from build123d import *

# Parameters (mm, degrees)
F0_W     = 30.4900507075
F0_H     = 16.8403594638
F0_R     = 3.175
F1_DEPTH = 25.4
F2_R     = 3.175
F3_DEPTH = 25.4
F4_DEPTH = 25.4


# Not quite as in the source:
# - a feature names something its author has since deleted; it is built from what else it names


with BuildPart() as f1:
    # F0 (on Front) → F1 (new body)
    with BuildSketch(Plane.XZ):
        Rectangle(F0_W, F0_H)
        with Locations((-7.6225126769, 0)):
            Circle(F0_R, mode=Mode.SUBTRACT)
        with Locations((7.6225126769, 0)):
            Circle(F0_R, mode=Mode.SUBTRACT)
        with Locations((-7.6225126769, 0)):
            Circle(F0_R)
        with Locations((7.6225126769, 0)):
            Circle(F0_R)
    extrude(amount=F1_DEPTH)

    # F2 (on face) → F3 (join)
    with BuildSketch(Plane(origin=(0, 0, 0), x_dir=(-1, 0, 0), z_dir=(0, 1, 0))):
        with Locations((10.1633502358, 0)):
            Circle(F2_R)
        with Locations((-10.1633502358, 0)):
            Circle(F2_R)
    extrude(amount=F3_DEPTH)

    # F4 (add): a face of the model
    f4_faces = [f1.faces().sort_by_distance(p)[0] for p in [
        (15.2450253537, -12.7, 0),
    ]]
    extrude(f4_faces, amount=F4_DEPTH)


solid = f1.part
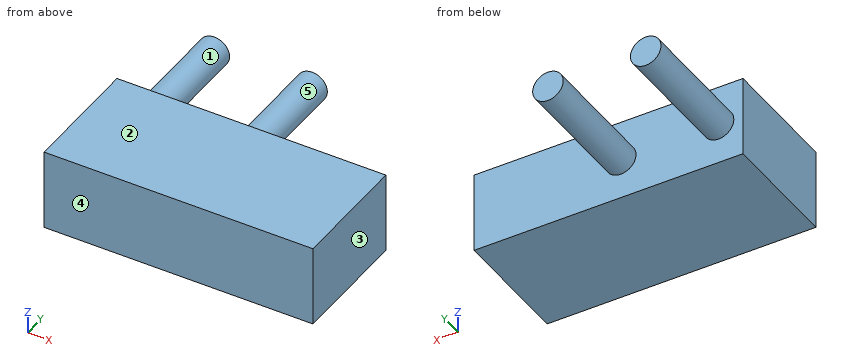
Check sheet for the modelled part. Datum: model origin and axes. Units: mm. Face numbers are marked on the shaded views. A direction names the side the tool comes from. Round coordinates to 2 decimals unless told otherwise and drop trailing zeros. Order: outer loops, then holes, each group sorted by start corner. A loop starts at its lowest first (then second) coordinate and runs counter-clockwise, first axis right, second up. Notation, with made-up numbers: M -7.75,-36.5 L 11.25,-36.5 A36 cw 11.25,1.5 Z; hole C 37,76 d8. An arc over 180 degrees is marked long. One line per item, written item: value. Start each with the question number.
1. Gauge pin test, flat ends, axial feed: P1, Ø12, axis at x = 15, y = 19.5, coming from the +Z side (3 decimals); P2, Ø3, axis at y = 19, z = 5.5, coming from the -X side; P3, Ø1, axis at y = 9.5, z = 3, coming from the -X side. Record the tip position at first contact, or that the pin passes through.
2. Scan lines: line 1 along Y through (x, z) = (-8, 5.25); line 2 along X through (y, z) = (2, -2.5); line 3 along X through (y, z) = (9, -0.5). Record each from-to range of solid material in increasing order.
3. Access from +Z, -Z, +X, -X, +Y, -Y to the whole of each face (thin tool, end or side, straight path). Record for the marked faces 1 and 2.
4. Section check A-A on z = 0. Enter the section's corners in (x, y).
5. Section check C-C on x = 30. Enter the section's corners in (y, z), and give its area (3 significant figures).
6. Section check B-B on y = 14. Enter the section's corners in (x, z) (3 decimals).
7. Release check for a two-part mould opening along X. For the marked faces 3, 4 and 5 record: released by +X, released by -X, zero draft, split by the parting line, or undercut.
8. Section check D-D on z = -5.25. Enter the section's corners in (x, y), and give its area (3 significant figures).
Results found:
1. P1: z = 3.175
1. P2: through
1. P3: x = -12.12
2. line 1: -25.4 to 0
2. line 2: -12.12 to -8.21, 8.21 to 12.12
2. line 3: -13.3 to -7.03, 7.03 to 13.3
3. face 1: +Y
3. face 2: +Z, +X, -X, +Y, -Y
4. outline: M -15.25,-25.4 L 40.65,-25.4 L 40.65,0 L 13.34,0 L 13.34,25.4 L 6.99,25.4 L 6.99,0 L -6.99,0 L -6.99,25.4 L -13.34,25.4 L -13.34,0 L -15.25,0 Z
5. outline: M -25.4,-8.42 L 0,-8.42 L 0,8.42 L -25.4,8.42 Z
5. area: 428 mm^2
6. outline: C -10.163,0 d6.35; C 10.163,0 d6.35
7. face 3: released by +X
7. face 4: zero draft
7. face 5: undercut
8. outline: M -15.25,-25.4 L 40.65,-25.4 L 40.65,0 L -15.25,0 Z
8. area: 1,420 mm^2
